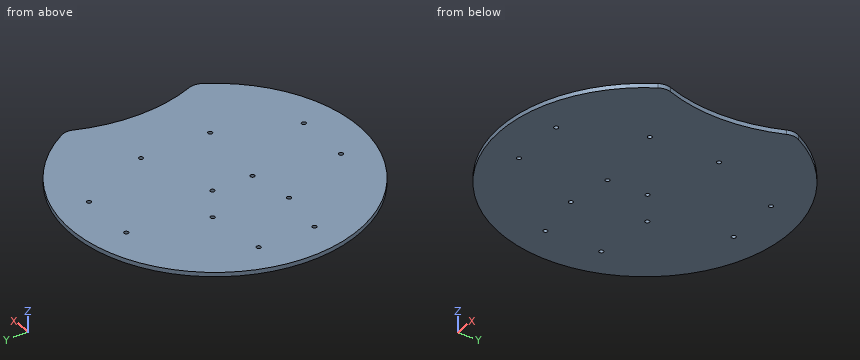
```python
from build123d import *

# Parameters (mm, degrees)
CROQUIS1_R              = 100
SALIENTE_EXTRUIR1_DEPTH = 3
CROQUIS3_R              = 110
CORTAR_EXTRUIR1_DEPTH   = 3
REDONDEO1_R             = 10
CROQUIS4_R              = 1.5
CORTAR_EXTRUIR2_DEPTH   = 142.453172607
CROQUIS5_R              = 1.5
CORTAR_EXTRUIR3_DEPTH   = 142.453172607


with BuildPart() as part:
    # Croquis1 → Saliente-Extruir1 (new body)
    with BuildSketch(Plane.XY):
        Circle(CROQUIS1_R)
    extrude(amount=SALIENTE_EXTRUIR1_DEPTH)

    # Croquis3 → Cortar-Extruir1 (cut)
    with BuildSketch(Plane.XY.offset(3)):
        with Locations((190, 0)):
            Circle(CROQUIS3_R)
    extrude(amount=-CORTAR_EXTRUIR1_DEPTH, mode=Mode.SUBTRACT)

    # Redondeo1
    redondeo1_edges = [part.edges().sort_by_distance(p)[0] for p in [
        (89.473684211, -44.659375654, 1.5),
        (89.473684211, 44.659375654, 1.5),
    ]]
    fillet(redondeo1_edges, radius=REDONDEO1_R)

    # Croquis4 → Cortar-Extruir2 (cut, through all)
    with BuildSketch(Plane.XY.offset(3)):
        with Locations((-33.815, 24.17)):
            Circle(CROQUIS4_R)
        with Locations((-41.315, -24.17)):
            Circle(CROQUIS4_R)
        with Locations((41.315, -24.17)):
            Circle(CROQUIS4_R)
        with Locations((41.315, 24.17)):
            Circle(CROQUIS4_R)
        with Locations((-10.31559482, -19.297497716)):
            Circle(CROQUIS4_R)
        with Locations((-10.311195262, 8.714642909)):
            Circle(CROQUIS4_R)
    extrude(amount=-CORTAR_EXTRUIR2_DEPTH, mode=Mode.SUBTRACT)

    # Croquis5 → Cortar-Extruir3 (cut, through all)
    with BuildSketch(Plane.XY.offset(3)):
        with Locations((-75, 19.5)):
            Circle(CROQUIS5_R)
        with Locations((-75, -19.5)):
            Circle(CROQUIS5_R)
        with Locations((19.5, 75)):
            Circle(CROQUIS5_R)
        with Locations((-19.5, 75)):
            Circle(CROQUIS5_R)
        with Locations((-19.5, -75)):
            Circle(CROQUIS5_R)
        with Locations((19.5, -75)):
            Circle(CROQUIS5_R)
    extrude(amount=-CORTAR_EXTRUIR3_DEPTH, mode=Mode.SUBTRACT)


solid = part.part
```
Geometry check sheet. Reference: the model listing, model coordinates, mm. Give positions to 0.01 mm unless a question says otherwise; leave off trailing zeros. Order: outer loops, then holes, each group sorted by start corner. A loop starts at its lowest first (then second) coordinate and runs counter-clockwise, first axis right, second up. Notation, with made-up numbers: (65, 87) -> (72, 87) arc R30 cw to (72, 113) -> close; hole circle Ø3 at (19, 50). An arc over 180 degrees is marked (long way). Write each question's results on one line, items separated by ' | '. Start each with the question number.
(1) Sectioned sample at C-C (y = -68). Enter the section's corners in (x, z), plus the area to 3 significant figures.
(2) Gauge pin test, flat ends, axial feed: P1, Ø2.5, axis at x = -41.315, y = -24.17, coming from the -Z side; P2, Ø4, axis at x = 19.5, y = -75, coming from the -Z side; P3, Ø1, axis at x = -14.5, z = 1.5, coming from the -Y side. Record the tip position at first contact, or that the pin passes through.
(3) Sectioned sample at A-A (z = 1.15). Give the number of separate pieces and of enclosed holes in the cut face, plus the area to 3 significant figures.
(4) Sectioned sample at B-B (x = 51). Enter the section's corners in (y, z), plus the area to 3 significant figures.
(5) Scan lines: line 1 (Y direction, x = 19.5, z = 1.9); line 2 (Y direction, x = -75, z = 2.1). Record each from-to range of solid material in increasing order.
Answer below:
1) outline: (-73.32, 0) -> (73.32, 0) -> (73.32, 3) -> (-73.32, 3) -> close | area: 440 mm2
2) P1: through | P2: z = 0 | P3: y = -99.02
3) separate pieces: 1 | enclosed holes: 12 | area: 30,100 mm2
4) outline: (-86.02, 0) -> (86.02, 0) -> (86.02, 3) -> (-86.02, 3) -> close | area: 516 mm2
5) line 1: -98.08 to -76.5, -73.5 to 73.5, 76.5 to 98.08 | line 2: -66.14 to -21, -18 to 18, 21 to 66.14
